Input: part model. Units: mm. Frame: model coordinates. Coordinates: 2 decimals unless noted, no trailing zeros. Use a Markdown table: item, result. Add a question column.
1. Section A-A on z = 2.15. State how many separate pieces and enclosed holes the cut face has, then the cut area to 3 significant figures.
2. Pin query (flat end, axial travel): pin 1 (0.8 mm diameter, centred on x = -9.23, y = -12.7, fed in from +Z); pin 2 (5 mm diameter, centred on x = -15, y = -1, fed in from -Z). Return the tip coordinate at first contact, or that it passes through.
3. Line query: L1, parallel to X at y = 12, z = 1.5 (3 decimals); L2, parallel to X at y = -36, z = 1.7 (3 decimals). Output: solid intervals per line, ascending. Write a range as [from, to].
4. Draft query along Y for faces 1 (the flat face through (-1, -47.625, 2)), 2 (the flat face through (-1, 47.625, 2)), 3 (the cylindrical face through (-14.645, 11.209, 1.565)). Return one class per face: +Y half, -Y half, draft (parallel to the pull), parting line (faces both ways), or undercut.
```python
from build123d import *

# Parameters (mm, degrees)
F0_W     = 95.25
F0_H     = 95.25
F0_R     = 2.4511
F1_DEPTH = 3.175
F2_R     = 0.635
F3_DEPTH = 5.08


with BuildPart() as f1:
    # F0 (on Top) → F1 (new body)
    with BuildSketch(Plane.XY):
        Rectangle(F0_W, F0_H)
        with Locations((-38.1, -38.1)):
            Circle(F0_R, mode=Mode.SUBTRACT)
        with Locations((-12.7, -38.1)):
            Circle(F0_R, mode=Mode.SUBTRACT)
        with Locations((-38.1, -12.7)):
            Circle(F0_R, mode=Mode.SUBTRACT)
        with Locations((-12.7, -12.7)):
            Circle(F0_R, mode=Mode.SUBTRACT)
        with Locations((12.7, -38.1)):
            Circle(F0_R, mode=Mode.SUBTRACT)
        with Locations((38.1, -38.1)):
            Circle(F0_R, mode=Mode.SUBTRACT)
        with Locations((12.7, -12.7)):
            Circle(F0_R, mode=Mode.SUBTRACT)
        with Locations((38.1, -12.7)):
            Circle(F0_R, mode=Mode.SUBTRACT)
        with Locations((-38.1, 12.7)):
            Circle(F0_R, mode=Mode.SUBTRACT)
        with Locations((-12.7, 12.7)):
            Circle(F0_R, mode=Mode.SUBTRACT)
        with Locations((-38.1, 38.1)):
            Circle(F0_R, mode=Mode.SUBTRACT)
        with Locations((-12.7, 38.1)):
            Circle(F0_R, mode=Mode.SUBTRACT)
        with Locations((12.7, 12.7)):
            Circle(F0_R, mode=Mode.SUBTRACT)
        with Locations((38.1, 12.7)):
            Circle(F0_R, mode=Mode.SUBTRACT)
        with Locations((12.7, 38.1)):
            Circle(F0_R, mode=Mode.SUBTRACT)
        with Locations((38.1, 38.1)):
            Circle(F0_R, mode=Mode.SUBTRACT)
    extrude(amount=F1_DEPTH)

    # F2 (on face) → F3 (cut)
    with BuildSketch(Plane.XY.offset(3.175)):
        with Locations((-41.5671, 38.1)):
            Circle(F2_R)
        with Locations((-38.1, 41.5671)):
            Circle(F2_R)
        with Locations((-34.6329, 38.1)):
            Circle(F2_R)
        with Locations((-41.5671, 12.7)):
            Circle(F2_R)
        with Locations((-38.1, 16.1671)):
            Circle(F2_R)
        with Locations((-34.6329, 12.7)):
            Circle(F2_R)
        with Locations((-41.5671, -12.7)):
            Circle(F2_R)
        with Locations((-38.1, -9.2329)):
            Circle(F2_R)
        with Locations((-34.6329, -12.7)):
            Circle(F2_R)
        with Locations((-41.5671, -38.1)):
            Circle(F2_R)
        with Locations((-38.1, -34.6329)):
            Circle(F2_R)
        with Locations((-34.6329, -38.1)):
            Circle(F2_R)
        with Locations((-16.1671, 38.1)):
            Circle(F2_R)
        with Locations((-12.7, 41.5671)):
            Circle(F2_R)
        with Locations((-9.2329, 38.1)):
            Circle(F2_R)
        with Locations((-16.1671, 12.7)):
            Circle(F2_R)
        with Locations((-12.7, 16.1671)):
            Circle(F2_R)
        with Locations((-9.2329, 12.7)):
            Circle(F2_R)
        with Locations((-16.1671, -12.7)):
            Circle(F2_R)
        with Locations((-12.7, -9.2329)):
            Circle(F2_R)
        with Locations((-9.2329, -12.7)):
            Circle(F2_R)
        with Locations((-16.1671, -38.1)):
            Circle(F2_R)
        with Locations((-12.7, -34.6329)):
            Circle(F2_R)
        with Locations((-9.2329, -38.1)):
            Circle(F2_R)
        with Locations((9.2329, 38.1)):
            Circle(F2_R)
        with Locations((12.7, 41.5671)):
            Circle(F2_R)
        with Locations((16.1671, 38.1)):
            Circle(F2_R)
        with Locations((9.2329, 12.7)):
            Circle(F2_R)
        with Locations((12.7, 16.1671)):
            Circle(F2_R)
        with Locations((16.1671, 12.7)):
            Circle(F2_R)
        with Locations((9.2329, -12.7)):
            Circle(F2_R)
        with Locations((12.7, -9.2329)):
            Circle(F2_R)
        with Locations((16.1671, -12.7)):
            Circle(F2_R)
        with Locations((9.2329, -38.1)):
            Circle(F2_R)
        with Locations((12.7, -34.6329)):
            Circle(F2_R)
        with Locations((16.1671, -38.1)):
            Circle(F2_R)
        with Locations((34.6329, 38.1)):
            Circle(F2_R)
        with Locations((38.1, 41.5671)):
            Circle(F2_R)
        with Locations((41.5671, 38.1)):
            Circle(F2_R)
        with Locations((34.6329, 12.7)):
            Circle(F2_R)
        with Locations((38.1, 16.1671)):
            Circle(F2_R)
        with Locations((41.5671, 12.7)):
            Circle(F2_R)
        with Locations((34.6329, -12.7)):
            Circle(F2_R)
        with Locations((38.1, -9.2329)):
            Circle(F2_R)
        with Locations((41.5671, -12.7)):
            Circle(F2_R)
        with Locations((34.6329, -38.1)):
            Circle(F2_R)
        with Locations((38.1, -34.6329)):
            Circle(F2_R)
        with Locations((41.5671, -38.1)):
            Circle(F2_R)
    extrude(amount=-F3_DEPTH, mode=Mode.SUBTRACT)


solid = f1.part
```
Answers below:
| question | item | result |
|---|---|---|
| 1 | separate pieces | 1 |
| 1 | enclosed holes | 64 |
| 1 | area | 8,710 mm² |
| 2 | pin 1 | passes through |
| 2 | pin 2 | stops at z = 0 |
| 3 | L1 | x = [-47.625, -40.449], [-35.751, -15.049], [-10.351, 10.351], [15.049, 35.751], [40.449, 47.625] |
| 3 | L2 | x = [-47.625, -39.364], [-36.836, -13.964], [-11.436, 11.436], [13.964, 36.836], [39.364, 47.625] |
| 4 | face 1 | -Y half |
| 4 | face 2 | +Y half |
| 4 | face 3 | undercut |
